Verification items for the finished model (mm, model axes). A direction names the side the tool comes from. Round coordinates to 2 decimals unless told otherwise and drop trailing zeros. Order: outer loops, then holes, each group sorted by start corner. A loop starts at its lowest first (then second) coordinate and runs counter-clockwise, first axis right, second up. Notation, with made-up numbers: M -13.75,1 L 0.25,1 A23 cw 0.25,15 Z; hole C -8.5,-20 d7. An arc over 180 degrees is marked long. Use CSV: the item, a comma, the result in double quotes. Start each with the question number.
Q1. Gauge pin test, flat ends, axial feed: pin 1 Ø1 at (x, z) = (-3.5, -77.5) entering from -Y; pin 2 Ø5 at (y, z) = (-4.5, -32) entering from +X; pin 3 Ø4.5 at (x, y) = (-3, -0.5) entering from +Z; pin 4 Ø12 at (y, z) = (5, -72.5) entering from +X. Record the tip position at first contact, or that the pin passes through.
Q2. Sectioned sample at A-A (z = -12.5). Enter the section's corners in (x, y).
Q3. Sectioned sample at B-B (z = -91). Enter the section's corners in (x, y), and give its area (3 significant figures).
Q4. Scan lines: line 1 (X direction, y = 9, z = -61); line 2 (Z direction, x = -4, y = 0.5); line 3 (Y direction, x = -2.5, z = -81.5). Record each from-to range of solid material in increasing order.
Q5. Mould release check, pull along Z, two halves, no side actions. Record for faces 3 (the face through (-1.495, -6.733, -35.234)), 4 (the face through (0, 0, -100)), 5 (the face through (3, -6, -17.005)), 6 (the face through (-0.88, -3.96, -41.99)): +Z half, -Z half, draft (parallel to the pull), parting line (faces both ways), or undercut.
Q6. Set-up check for faces 1 (the face through (-2.57, -11.57, -77.04)), 2 (the face through (5, 1.6, -10.9)): record each of +Z, -Z, +X, -X, +Y, -Y from which the full face is reachable in a straight line by a thin tool's end or side.
```python
from build123d import *


with BuildPart() as f1:
    # F0 (on Front) → F1 (revolve)
    with BuildSketch(Plane.XZ):
        with BuildLine():
            Line((5.250814, -16.005392), (5.250814, -6.005392))
            Line((5.250814, -6.005392), (0, -2.836546))
            Line((0, -2.836546), (0, -100))
            Line((0, -100), (11.851529, -100))
            Line((11.851529, -100), (11.851529, -54.711972))
            ThreePointArc((11.851529, -54.711972), (10.504539, -51.460051), (7.252618, -50.113061))
            ThreePointArc((7.252618, -50.113061), (3.472311, -48.622302), (2.947314, -44.592729))
            Line((2.947314, -44.592729), (6.841612, -35.464703))
            Line((6.841612, -35.464703), (7.723922, -31.773916))
            Line((7.723922, -31.773916), (7.723922, -17.005392))
            Line((7.723922, -17.005392), (6.250814, -17.005392))
            ThreePointArc((6.250814, -17.005392), (5.543708, -16.712499), (5.250814, -16.005392))
        make_face()
    revolve(axis=Axis((0, 0, -51.418273), (0, 0, 1)))


solid = f1.part
```
Verdict:
1,pin 1,"stops at y = -11.47"
1,pin 2,"stops at x = 7.46"
1,pin 3,"stops at z = -3.31"
1,pin 4,"stops at x = 11.85"
2,outline,"C 0,0 d10.5"
3,outline,"C 0,0 d23.7"
3,area,"441 mm²"
4,line 1,"x = -7.71 to 7.71"
4,line 2,"z = -100 to -49.21, -42.05 to -5.27"
4,line 3,"y = -11.58 to 11.58"
5,face 3,"undercut"
5,face 4,"-Z half"
5,face 5,"+Z half"
5,face 6,"undercut"
6,face 1,"+Z, -Z"
6,face 2,"+Z"
